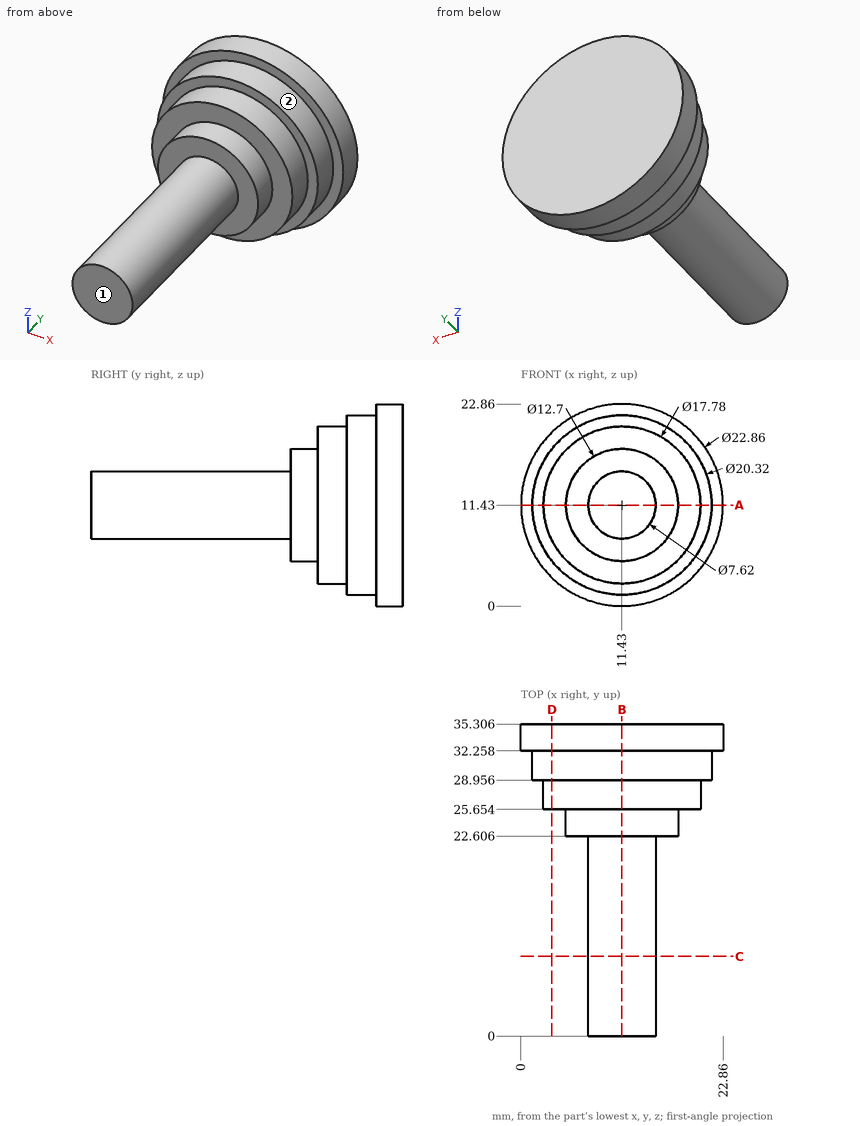
Print and shaded views of the part. All mm, measured from the part's lowest x, y and z. A direction names the side the tool comes from. Round coordinates to 2 decimals unless told otherwise and drop trailing zeros. Write each loop counter-clockwise with the first axis right and the second up, starting at its lowest first coordinate (ties: lowest second). Pieces come first, ordered by that corner, then holes.
Item 1: Drop flat-ended pins along their axis: pin 1 Ø10 at (x, y) = (11.5, 22.5) entering from -Z; pin 2 Ø10 at (y, z) = (17, 13.5) entering from -X; pin 3 Ø1.5 at (x, z) = (20, 20) entering from -Y. Give the stop position or say it passes through.
Results:
pin 1: stops at z = 2.54
pin 2: stops at x = 7.62
pin 3: stops at y = 32.26
Item 2: Cut at B-B, the plane x = 11.43. Give the cut face in (y, z), plus the area to 3 significant figures.
Results:
outline: (0, 7.62) - (22.61, 7.62) - (22.61, 5.08) - (25.65, 5.08) - (25.65, 2.54) - (28.96, 2.54) - (28.96, 1.27) - (32.26, 1.27) - (32.26, 0) - (35.31, 0) - (35.31, 22.86) - (32.26, 22.86) - (32.26, 21.59) - (28.96, 21.59) - (28.96, 20.32) - (25.65, 20.32) - (25.65, 17.78) - (22.61, 17.78) - (22.61, 15.24) - (0, 15.24) - close
area: 406 mm2
Item 3: Which spindle directions (+Z, -Z, +X, -X, +Y, -Y) get a long thin tool onto all of the face, cutting with end or side? Do the marked faces 1 and 2. Say none if no direction does.
Results:
face 1: +Z, -Z, +X, -X, -Y
face 2: -Y
Item 4: Cut at A-A, the plane z = 11.43. Give the cut face in (x, y).
Results:
outline: (0, 32.26) - (1.27, 32.26) - (1.27, 28.96) - (2.54, 28.96) - (2.54, 25.65) - (5.08, 25.65) - (5.08, 22.61) - (7.62, 22.61) - (7.62, 0) - (15.24, 0) - (15.24, 22.61) - (17.78, 22.61) - (17.78, 25.65) - (20.32, 25.65) - (20.32, 28.96) - (21.59, 28.96) - (21.59, 32.26) - (22.86, 32.26) - (22.86, 35.31) - (0, 35.31) - close
Item 5: Cut at C-C, the plane y = 9. Give the cut face in (x, z), plus the area to 3 significant figures.
Results:
outline: circle Ø7.62 at (11.43, 11.43)
area: 45.6 mm2
Item 6: Probe L1, parallel to Y at x = 19.25, z = 4; L2, parallel to Y at x = 21, z = 10.25; L3, parallel to Z at x = 11.5, y = 5. List the from-to ranges inside material, lowest first.
Results:
L1: y = 32.26 to 35.31
L2: y = 28.96 to 35.31
L3: z = 7.62 to 15.24
Item 7: Cut at D-D, the plane x = 3.5. Give the cut face in (y, z).
Results:
outline: (25.65, 7.41) - (28.96, 7.41) - (28.96, 5.08) - (32.26, 5.08) - (32.26, 3.2) - (35.31, 3.2) - (35.31, 19.66) - (32.26, 19.66) - (32.26, 17.78) - (28.96, 17.78) - (28.96, 15.45) - (25.65, 15.45) - close
